CAD build for the part. Positions are in the model's coordinates, mm. A direction names the side the tool comes from. Give positions to 0.01 mm unless a question says otherwise; leave off trailing zeros. Write each loop counter-clockwise with the first axis right and the second up, starting at its lowest first coordinate (ties: lowest second). Pieces come first, ordered by that corner, then holes. Notation, with made-up numbers: (76, 75) -> (114, 75) arc R24 cw to (114, 112) -> close; hole circle Ø3 at (-37.5, 32.25). An arc over 180 degrees is marked (long way). Answer in a Markdown table with one row per item. Add a question column.
```python
from build123d import *

# Parameters (mm, degrees)
SKETCH_R        = 12
SKETCH_R_2      = 1.7
PAD_DEPTH       = 24.5
POCKET_DEPTH    = 19.5
POCKET001_DEPTH = 64.001
POCKET002_DEPTH = 225.811705
SKETCH004_R     = 2.6
POCKET003_DEPTH = 225.811705
FILLET_R        = 1


with BuildPart() as part:
    # Sketch → Pad (new body)
    with BuildSketch(Plane.XY):
        Polygon((-26.5, -21), (26.5, -21), (26.5, 17), (37.5, 17), (37.5, 22), (26.5, 22), (26.5, 41.5), (-26.5, 41.5), (-26.5, 22), (-37.5, 22), (-37.5, 17), (-26.5, 17), align=None)
        Circle(SKETCH_R, mode=Mode.SUBTRACT)
        with Locations((-15.5, 15.5)):
            Circle(SKETCH_R_2, mode=Mode.SUBTRACT)
        with Locations((15.5, 15.5)):
            Circle(SKETCH_R_2, mode=Mode.SUBTRACT)
        with Locations((-15.5, -15.5)):
            Circle(SKETCH_R_2, mode=Mode.SUBTRACT)
        with Locations((15.5, -15.5)):
            Circle(SKETCH_R_2, mode=Mode.SUBTRACT)
    extrude(amount=PAD_DEPTH)

    # Sketch001 (on Face18 of Pad) → Pocket (cut)
    with BuildSketch(Plane(origin=(0, 0, 0), x_dir=(1, 0, 0), z_dir=(0, 0, -1))):
        Polygon((-26.5, -41.5), (26.5, -41.5), (26.5, -22), (21.5, -22), (21.5, 21), (-21.5, 21), (-21.5, -22), (-26.5, -22), align=None)
    extrude(amount=-POCKET_DEPTH, mode=Mode.SUBTRACT)

    # Sketch002 (on Face7 of Pocket) → Pocket001 (cut, through all)
    with BuildSketch(Plane.YZ.offset(26.5)):
        Polygon((17, 0), (-21, 0), (-21, 19.5), align=None)
    extrude(amount=-POCKET001_DEPTH, mode=Mode.SUBTRACT)

    # Sketch003 (on Face6 of Pocket001) → Pocket002 (cut, through all)
    with BuildSketch(Plane.XY.offset(24.5)):
        with BuildLine():
            Line((-26.5, 34.6), (-20, 34.6))
            ThreePointArc((-20, 29.4), (-17.4, 32), (-20, 34.6))
            Line((-20, 29.4), (-26.5, 29.4))
            Line((-26.5, 29.4), (-26.5, 34.6))
        make_face()
    pocket002 = extrude(amount=-POCKET002_DEPTH, mode=Mode.SUBTRACT)

    # Sketch004 (on Face27 of Pocket002) → Pocket003 (cut, through all)
    with BuildSketch(Plane.XZ.offset(-17)):
        with Locations((-32, 9.5)):
            Circle(SKETCH004_R)
    pocket003 = extrude(amount=-POCKET003_DEPTH, mode=Mode.SUBTRACT)

    # Mirrored: Pocket003 across Sketch004 V_Axis
    add(pocket003.mirror(Plane(origin=(0, 17, 0), x_dir=(0, -1, 0), z_dir=(1, 0, 0))), mode=Mode.SUBTRACT)

    # Mirrored001: Pocket002 across Sketch003 V_Axis
    add(pocket002.mirror(Plane(origin=(0, 0, 24.5), x_dir=(0, 0, 1), z_dir=(1, 0, 0))), mode=Mode.SUBTRACT)

    # Fillet
    fillet_edges = [part.edges().sort_by_distance(p)[0] for p in [
        (-26.5, 41.5, 22),
        (-26.5, 34.6, 22),
        (-26.5, 29.4, 22),
        (26.5, 34.6, 22),
        (26.5, 41.5, 22),
        (26.5, 29.4, 22),
        (-26.5, -21, 22),
        (26.5, -21, 22),
        (-21.5, 22, 9.75),
        (21.5, 22, 9.75),
        (-37.5, 19.5, 24.5),
        (37.5, 19.5, 24.5),
        (-37.5, 19.5, 0),
        (37.5, 19.5, 0),
    ]]
    fillet(fillet_edges, radius=FILLET_R)


solid = part.part
```
Item 1: Drop flat-ended pins along their axis: pin 1 Ø2 at (y, z) = (9, 15.5) entering from +X; pin 2 Ø3 at (x, y) = (-15.5, -15.5) entering from -Z; pin 3 Ø8.5 at (x, z) = (32, 9.5) entering from +Y; pin 4 Ø7 at (x, z) = (-32, 9.5) entering from -Y. Give the stop position or say it passes through.
Item 2: Slice it at B-B, the plane x = 15.5. List the corners of the cut face in (y, z).
Item 3: Mould opens along X. For faces 5 (the face through (-26.5, 25, 22)), 6 (the face through (17.07, -16.15, 21.96)), 7 (the face through (0, -21, 22)) say: released by +X, released by -X, zero draft, split by the parting line, or undercut.
Item 4: Probe L1, parallel to Y at x = 15.5, z = 23.1; L2, parallel to X at y = -9, z = 19; L3, parallel to X at y = 15.5, z = 22.8. List the from-to ranges inside material, lowest first. Write a range as from..to.
Item 5: Which spindle directions (+Z, -Z, +X, -X, +Y, -Y) get a long thin tool onto all of the face, cutting with end or side? Do faces 1 (the face through (-21.5, 4, 12)), 2 (the face through (-23, 29.4, 22)), 3 (the face through (26.5, 2, 15)), 4 (the face through (26.5, 38, 22)). Say none if no direction does.
Item 6: Slice it at D-D, the plane y = -5. List the corners of the cut face in (x, z), then the cut area to 3 significant figures.
Item 7: Slice it at C-C, the plane y = 15.5. List the corners of the cut face in (x, z), then the cut area to 3 significant figures.
Item 8: Slice it at A-A, the plane x = 0. List the corners of the cut face in (y, z), then the cut area to 4 significant figures.
Answer key:
| question | item | result |
|---|---|---|
| 1 | pin 1 | stops at x = 26.5 |
| 1 | pin 2 | passes through |
| 1 | pin 3 | stops at y = 22 |
| 1 | pin 4 | stops at y = 17 |
| 2 | outline | (-21, 19.5) -> (-17.2, 19.5) -> (-17.2, 24.5) -> (-21, 24.5) -> close; (-13.8, 19.5) -> (13.8, 19.5) -> (13.8, 24.5) -> (-13.8, 24.5) -> close; (17.2, 19.5) -> (41.5, 19.5) -> (41.5, 24.5) -> (17.2, 24.5) -> close |
| 3 | face 5 | released by -X |
| 3 | face 6 | undercut |
| 3 | face 7 | zero draft |
| 4 | L1 | y = -21..-17.2, -13.8..13.8, 17.2..41.5 |
| 4 | L2 | x = -26.5..-21.5, 21.5..26.5 |
| 4 | L3 | x = -26.5..-17.2, -13.8..13.8, 17.2..26.5 |
| 5 | face 1 | -Z, +Y, -Y |
| 5 | face 2 | +Z, -Z, -X |
| 5 | face 3 | +Z, -Z, +X, -Y |
| 5 | face 4 | +Z, -Z, +X, +Y |
| 6 | outline | (-26.5, 11.29) -> (-21.5, 11.29) -> (-21.5, 19.5) -> (-10.91, 19.5) -> (-10.91, 24.5) -> (-26.5, 24.5) -> close; (10.91, 19.5) -> (21.5, 19.5) -> (21.5, 11.29) -> (26.5, 11.29) -> (26.5, 24.5) -> (10.91, 24.5) -> close |
| 6 | area | 238 mm² |
| 7 | outline | (-26.5, 0.77) -> (-21.5, 0.77) -> (-21.5, 19.5) -> (-17.2, 19.5) -> (-17.2, 24.5) -> (-26.5, 24.5) -> close; (-13.8, 19.5) -> (13.8, 19.5) -> (13.8, 24.5) -> (-13.8, 24.5) -> close; (17.2, 19.5) -> (21.5, 19.5) -> (21.5, 0.77) -> (26.5, 0.77) -> (26.5, 24.5) -> (17.2, 24.5) -> close |
| 7 | area | 418 mm² |
| 8 | outline | (-21, 19.5) -> (-12, 19.5) -> (-12, 24.5) -> (-21, 24.5) -> close; (12, 19.5) -> (41.5, 19.5) -> (41.5, 24.5) -> (12, 24.5) -> close |
| 8 | area | 192.5 mm² |
